from build123d import *

# Parameters (mm, degrees)
SKETCH1_W           = 89
SKETCH1_H           = 89
SKETCH1_W_2         = 83
SKETCH1_H_2         = 83
BOSS_EXTRUDE1_DEPTH = 2
SKETCH4_W           = 6
SKETCH4_H           = 6
SKETCH4_R           = 1.7
BOSS_EXTRUDE3_DEPTH = 4
FILLET3_R           = 3
FILLET4_R           = 3


with BuildPart() as part:
    # Sketch1 → Boss-Extrude1 (new body, symmetric)
    with BuildSketch(Plane(origin=(0, 0, 0), x_dir=(1, 0, 0), z_dir=(0, 1, 0))):
        with Locations((44.5, 44.5)):
            Rectangle(SKETCH1_W, SKETCH1_H)
        with Locations((44.5, 44.5)):
            Rectangle(SKETCH1_W_2, SKETCH1_H_2, mode=Mode.SUBTRACT)
    extrude(amount=BOSS_EXTRUDE1_DEPTH, both=True)

    # Sketch4 → Boss-Extrude3 (add)
    with BuildSketch(Plane.XZ.offset(2)):
        with Locations((83, -6)):
            Rectangle(SKETCH4_W, SKETCH4_H)
        with Locations((83, -6)):
            Circle(SKETCH4_R, mode=Mode.SUBTRACT)
        with Locations((6, -6)):
            Rectangle(SKETCH4_W, SKETCH4_H)
        with Locations((6, -6)):
            Circle(SKETCH4_R, mode=Mode.SUBTRACT)
        with Locations((83, -83)):
            Rectangle(SKETCH4_W, SKETCH4_H)
        with Locations((83, -83)):
            Circle(SKETCH4_R, mode=Mode.SUBTRACT)
        with Locations((6, -83)):
            Rectangle(SKETCH4_W, SKETCH4_H)
        with Locations((6, -83)):
            Circle(SKETCH4_R, mode=Mode.SUBTRACT)
    extrude(amount=-BOSS_EXTRUDE3_DEPTH)

    # Fillet3
    fillet3_edges = [part.edges().sort_by_distance(p)[0] for p in [
        (9, 0, -9),
        (80, 0, -9),
        (9, 0, -80),
        (80, 0, -80),
    ]]
    fillet(fillet3_edges, radius=FILLET3_R)

    # Fillet4
    fillet4_edges = [part.edges().sort_by_distance(p)[0] for p in [
        (0, 0, -89),
        (89, 0, -89),
        (89, 0, 0),
        (0, 0, 0),
    ]]
    fillet(fillet4_edges, radius=FILLET4_R)


solid = part.part
Input: part model. Units: mm. Frame: model coordinates. A direction names the side the tool comes from. Coordinates: 2 decimals unless noted, no trailing zeros. Order: outer loops, then holes, each group sorted by start corner. A loop starts at its lowest first (then second) coordinate and runs counter-clockwise, first axis right, second up. Notation, with made-up numbers: M -12.5,28 L -6.5,28 A8 cw -6.5,33 Z; hole C 1.25,88.5 d4. An arc over 180 degrees is marked long. One line per question, with ' | ' between items.
Item 1: Section C-C (y = 0.5). Output: boundary loops of the cut face in (x, z).
Geometry results:
outline: M 0,-86 A3 ccw 3,-89 L 86,-89 A3 ccw 89,-86 L 89,-3 A3 ccw 86,0 L 3,0 A3 ccw 0,-3 Z; hole M 3,-80 L 6,-80 A3 cw 9,-83 L 9,-86 L 80,-86 L 80,-83 A3 cw 83,-80 L 86,-80 L 86,-9 L 83,-9 A3 cw 80,-6 L 80,-3 L 9,-3 L 9,-6 A3 cw 6,-9 L 3,-9 Z; hole C 6,-83 d3.4; hole C 6,-6 d3.4; hole C 83,-83 d3.4; hole C 83,-6 d3.4
Item 2: Section B-B (x = 40). Output: boundary loops of the cut face in (y, z).
Geometry results:
outline: M -2,-89 L 2,-89 L 2,-86 L -2,-86 Z; M -2,-3 L 2,-3 L 2,0 L -2,0 Z
Item 3: Reachability of faces 5 (the flat face through (44, -2, -1)), 6 (the cylindrical face through (80.86, 0.03, -8.1)) from +Z, -Z, +X, -X, +Y, -Y: full face, straight path, thin tool, end or side. Return the list, or none.
Geometry results:
face 5: +Z, -Z, +X, -X, -Y | face 6: +Y, -Y
Item 4: Ray query, line 1 along Z through (x, y) = (6, 0.8); line 2 along X through (y, z) = (1.25, -83); line 3 along X through (y, z) = (1.8, -51). Return the intervals inside material, ascending.
Geometry results:
line 1: z = -89 to -84.7, -81.3 to -80, -9 to -7.7, -4.3 to 0 | line 2: x = 0 to 4.3, 7.7 to 9, 80 to 81.3, 84.7 to 89 | line 3: x = 0 to 3, 86 to 89
Item 5: Draft query along Z for faces 1 (the cylindrical face through (0.86, -0.03, -88.1)), 2 (the flat face through (44, 2, -1)), 3 (the cylindrical face through (0.86, 0.03, -0.9)), 4 (the flat face through (84, 0, -9)). Return one class per face: released by +Z, released by -Z, zero draft, split by the parting line, or undercut.
Geometry results:
face 1: released by -Z | face 2: zero draft | face 3: released by +Z | face 4: undercut
Item 6: Pin query (flat end, axial travel): pin 1 (5.5 mm diameter, centred on x = 83, z = -6, fed in from -Y). Return the tip coordinate at first contact, or that it passes through.
Geometry results:
pin 1: stops at y = -2
Item 7: Section A-A (z = -48). Output: boundary loops of the cut face in (x, y).
Geometry results:
outline: M 0,-2 L 3,-2 L 3,2 L 0,2 Z; M 86,-2 L 89,-2 L 89,2 L 86,2 Z
